```python
from build123d import *

# Parameters (mm, degrees)
F0_R          = 9
F1_DEPTH      = 20
F3_DEPTH      = 5
F3_DEPTH_BACK = 25


with BuildPart() as f1:
    # F0 (on Top) → F1 (new body)
    with BuildSketch(Plane.XY):
        Circle(F0_R)
    extrude(amount=F1_DEPTH)

    # F2 (on Front) → F3 (cut, two sides)
    with BuildSketch(Plane.XZ) as f3_sk:
        Polygon((6, 18), (4, 18), (4, 10), (9, 10), (9, 20), (6, 20), align=None)
        Polygon((-6, 18), (-6, 20), (-9, 20), (-9, 10), (-4, 10), (-4, 18), align=None)
    extrude(amount=-F3_DEPTH, mode=Mode.SUBTRACT)
    extrude(f3_sk.sketch, amount=F3_DEPTH_BACK, mode=Mode.SUBTRACT)


solid = f1.part
```
Build history of the part. All positions in model axes, mm. A direction names the side the tool comes from. Give positions to 0.01 mm unless a question says otherwise; leave off trailing zeros. Loops run counter-clockwise (first coordinate to the right, second up) from the corner with the lowest first, then second, coordinate; pieces in that order, holes last. Notation, with made-up numbers: (86, -12.75) -> (98, -12.75) arc R10 cw to (98, -7.75) -> close; hole circle Ø8 at (38.5, 69.5). An arc over 180 degrees is marked (long way). One line per question, with ' | ' between items. Start each with the question number.
1) Probe L1, parallel to Z at x = -5, y = -7.25; L2, parallel to Z at x = -6.5, y = 0.75; L3, parallel to X at y = -0.75, z = 19. List the from-to ranges inside material, lowest first.
2) Cut at C-C (x = 4.75). Give the cut face in (y, z), plus the area to 3 significant figures.
3) Pin check, flat tips, straight feed: pin 1 (2 mm diameter, centred on y = -3, z = 18.5, fed in from -X); pin 2 (1 mm diameter, centred on x = 5.5, z = 13, fed in from -Y); pin 3 (2 mm diameter, centred on x = -5, z = 10, fed in from +Y); pin 4 (0.6 mm diameter, centred on x = -5.5, y = -1, fed in from -Z). Stop position of each tip, or through.
4) 3-axis set-ups, long thin cutter, end or side, ignore diameter. For faces 1 (the flat face through (5, -1, 18)), 2 (the flat face through (6, -1, 19)), 3 (the flat face through (-5, -1, 18)), 4 (the cylindrical face through (-1.172, 8.923, 7.638)): which of +Z, -Z, +X, -X, +Y, -Y reach the whole face in a straight line?
5) Cut at A-A (y = 0). Give the cut face in (x, z).
6) Cut at B-B (z = 7.5). Give the cut face in (x, y), plus the area to 3 significant figures.
7) Cut at D-D (y = -5.25). Give the cut face in (x, z), plus the area to 3 significant figures.
8) Two-plate mould, pull along Z, no slides. Class faces 5 (the flat face through (0, 0, 20)), 6 (the flat face through (6, 0, 10)), 7 (the flat face through (0, 0, 0)), 8 (the flat face through (-6, -1, 19)): released by +Z, released by -Z, zero draft, split by the parting line, or undercut.
Return value:
1) L1: 0 to 10, 18 to 20 | L2: 0 to 10 | L3: -6 to 6
2) outline: (-7.64, 0) -> (7.64, 0) -> (7.64, 20) -> (-7.64, 20) -> (-7.64, 18) -> (5, 18) -> (5, 10) -> (-7.64, 10) -> close | area: 205 mm^2
3) pin 1: x = -6 | pin 2: y = 5 | pin 3: y = 8.06 | pin 4: z = 0
4) face 1: +X, -Y | face 2: +Z, +X, -Y | face 3: -X, -Y | face 4: +Z, -Z
5) outline: (-9, 0) -> (9, 0) -> (9, 10) -> (4, 10) -> (4, 18) -> (6, 18) -> (6, 20) -> (-6, 20) -> (-6, 18) -> (-4, 18) -> (-4, 10) -> (-9, 10) -> close
6) outline: circle Ø18 at (0, 0) | area: 254 mm^2
7) outline: (-7.31, 0) -> (7.31, 0) -> (7.31, 10) -> (4, 10) -> (4, 18) -> (6, 18) -> (6, 20) -> (-6, 20) -> (-6, 18) -> (-4, 18) -> (-4, 10) -> (-7.31, 10) -> close | area: 234 mm^2
8) face 5: released by +Z | face 6: undercut | face 7: released by -Z | face 8: zero draft
